Answer from the drawing. Dimensions are ordinates in mm from the lowest x, y and z of the part. A direction names the side the tool comes from. Give positions to 0.01 mm unless a question says otherwise; leave off trailing zeros. Loops run counter-clockwise (first coordinate to the right, second up) from the corner with the lowest first, then second, coordinate; pieces in that order, holes last. Notation, with made-up numbers: (17.5, 26.25) - (73.5, 26.25) arc R27 ccw to (73.5, 58.25) - close; hole circle Ø7 at (12, 26). An arc over 180 degrees is marked (long way). One line per question, with ' | ' between items. Start each with the question number.
1. This flat-tipped pin is pushed along its axis until it touches: pin 1 (2 mm diameter, centred on y = 1.5, z = 2, fed in from +X). Where does it stop, or does it pass through?
2. Section C-C (z = 2.25) is taken. Determine the outline of the cut face in (x, y).
3. Find the intervals of material crossed by line 1 (Z direction, x = 0.8, y = 3.85); line 2 (Y direction, x = 3, z = 2.25); line 3 (Y direction, x = 1.85, z = 6.25), in increasing order.
4. Section D-D (y = 4) is taken. Determine the outline of the cut face in (x, z), plus the area to 3 significant figures.
5. Section B-B (x = 3.4) is taken. Determine the outline of the cut face in (y, z).
6. For a pull along Y with two mould halves and no side action, classify the marked faces 3, 4 and 5 as released by +Y, released by -Y, zero draft, split by the parting line, or undercut.
7. Which of the six approach directions +Z, -Z, +X, -X, +Y, -Y give full straight-line access (tool end or side, diameter ignored) to the marked faces 1 and 2?
8. Section A-A (y = 1.9) is taken. Determine the outline of the cut face in (x, z).
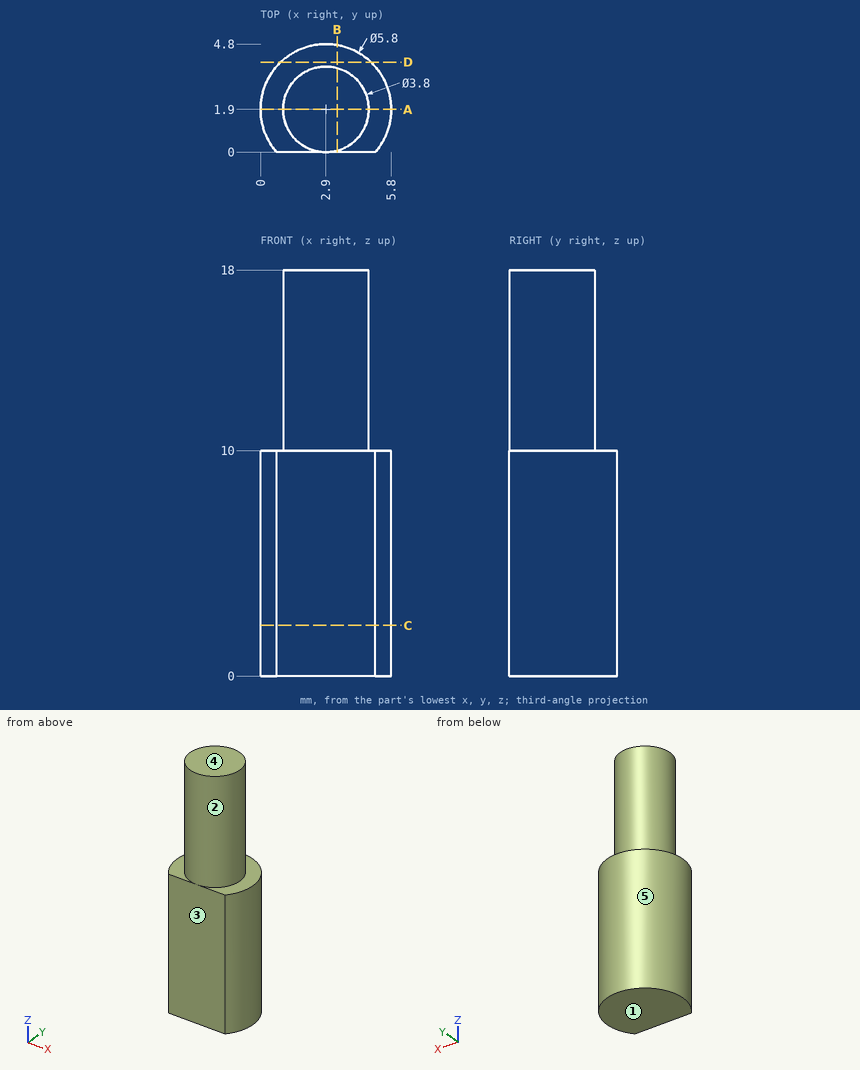
Conclusion:
1) pin 1: x = 5.8
2) outline: (0.71, 0) - (5.09, 0) arc R2.9 ccw (long way) to start
3) line 1: 0 to 10 | line 2: 0 to 4.8 | line 3: 0 to 4.6
4) outline: (0.9, 0) - (4.9, 0) - (4.9, 10) - (0.9, 10) - close | area: 40.0 mm²
5) outline: (0, 0) - (4.76, 0) - (4.76, 10) - (3.73, 10) - (3.73, 18) - (0.07, 18) - (0.07, 10) - (0, 10) - close
6) face 3: released by -Y | face 4: zero draft | face 5: split by the parting line
7) face 1: -Z, +X, -X, +Y, -Y | face 2: +Z
8) outline: (0, 0) - (5.8, 0) - (5.8, 10) - (4.8, 10) - (4.8, 18) - (1, 18) - (1, 10) - (0, 10) - close
